Check sheet for the drawn part. Datum: minimum x, y, z corner. Units: mm. A direction names the side the tool comes from. Give positions to 0.01 mm unless a question says otherwise; leave off trailing zeros. Order: outer loops, then holes, each group sorted by start corner. A loop starts at its lowest first (then second) coordinate and runs counter-clockwise, first axis right, second up.
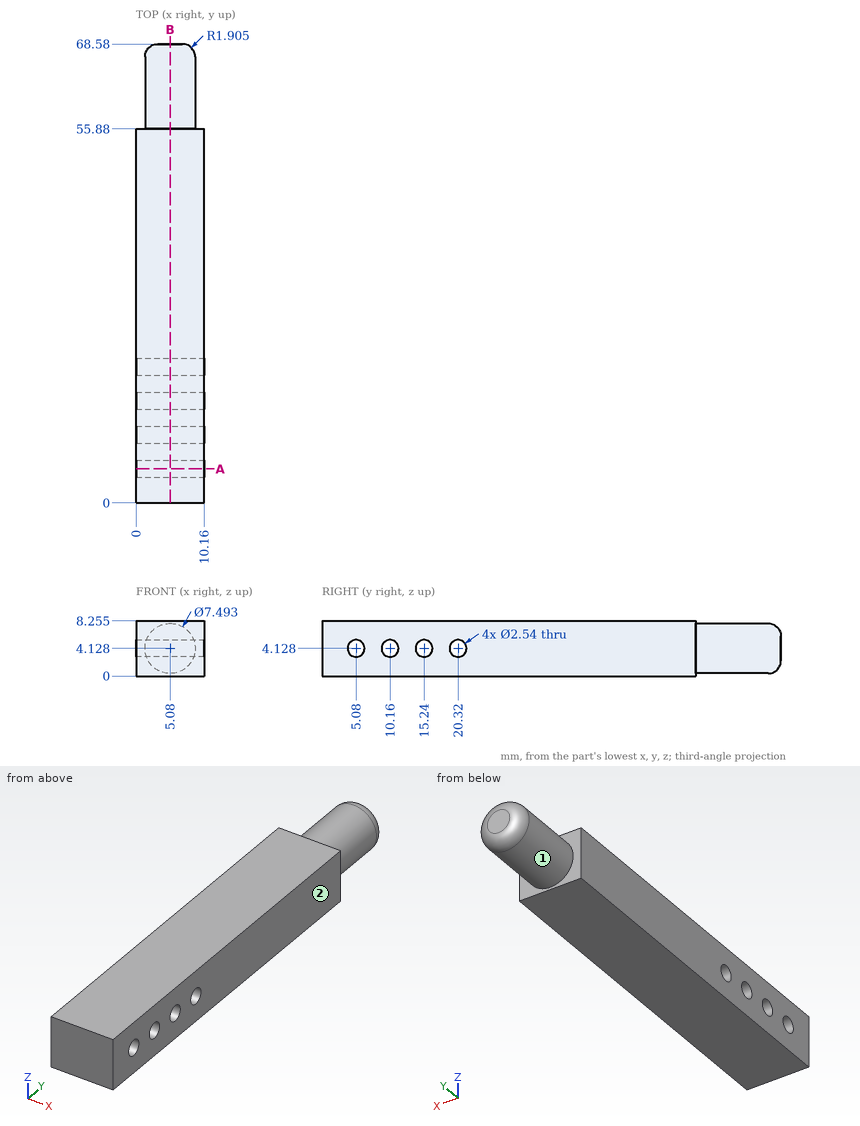
(1) Go/stop test with flat-tipped pins: pin 1 (1.5 mm diameter, centred on x = 2, y = 11.5, fed in from -Z); pin 2 (2 mm diameter, centred on x = 9, z = 5, fed in from +Y) (1 decimal); pin 3 (1.5 mm diameter, centred on y = 5.08, z = 4.13, fed in from +X). Record where each tip stops, or that it passes through.
Solved:
pin 1: stops at z = 0
pin 2: stops at y = 68.2
pin 3: passes through
(2) Section check B-B, the plane x = 5.08. Give the number of separate pieces and of enclosed holes in the cut face.
Solved:
separate pieces: 1
enclosed holes: 4
(3) Section check A-A, the plane y = 5.08. Enter the section's corners in (x, z) (1 decimal).
Solved:
outline: (0, 0) - (10.2, 0) - (10.2, 2.9) - (0, 2.9) - close; (0, 5.4) - (10.2, 5.4) - (10.2, 8.3) - (0, 8.3) - close
(4) Scan lines: line 1 (Z direction, x = 2, y = 10) (1 decimal); line 2 (Y direction, x = 0.75, z = 4); line 3 (Y direction, x = 3, z = 4.5) (1 decimal). Record each from-to range of solid material in increasing order.
Solved:
line 1: z = 0 to 2.9, 5.4 to 8.3
line 2: y = 0 to 3.82, 6.34 to 8.9, 11.42 to 13.98, 16.5 to 19.06, 21.58 to 55.88
line 3: y = 0 to 3.9, 6.3 to 8.9, 11.4 to 14, 16.5 to 19.1, 21.5 to 68.6
(5) Set-up check for the marked faces 1 and 2: record each of +Z, -Z, +X, -X, +Y, -Y from which the full face is reachable in a straight line by a thin tool's end or side.
Solved:
face 1: +Y
face 2: +Z, -Z, +X, +Y, -Y
